```python
from build123d import *

# Parameters (mm, degrees)
BOSS_EXTRUDE1_DEPTH = 12.7
BOSS_EXTRUDE2_DEPTH = 127
BOSS_EXTRUDE3_START = -12.7
SKETCH2_R           = 38.1
SKETCH2_R_2         = 31.75
BOSS_EXTRUDE3_DEPTH = 12.7
BOSS_EXTRUDE4_START = 76.2
BOSS_EXTRUDE4_DEPTH = 76.2


with BuildPart() as part:
    # Sketch1 → Boss-Extrude1 (new body)
    with BuildSketch(Plane(origin=(0, 0, 0), x_dir=(1, 0, 0), z_dir=(0, 1, 0))):
        with BuildLine():
            ThreePointArc((-38.1, 0), (-32.995567884, -19.05), (-19.05, -32.995567884))
            Line((-19.05, -32.995567884), (-15.875, -27.49630657))
            ThreePointArc((-15.875, -27.49630657), (-27.49630657, -15.875), (-31.75, 0))
            Line((-31.75, 0), (-38.1, 0))
        make_face()
        with BuildLine():
            ThreePointArc((-32.995567884, 19.05), (-36.801773982, 9.861005618), (-38.1, 0))
            Line((-38.1, 0), (-31.75, 0))
            ThreePointArc((-31.75, 0), (-30.668144985, 8.217504682), (-27.49630657, 15.875))
            Line((-27.49630657, 15.875), (-32.995567884, 19.05))
        make_face()
        with BuildLine():
            ThreePointArc((0, 38.1), (-19.05, 32.995567884), (-32.995567884, 19.05))
            Line((-32.995567884, 19.05), (-27.49630657, 15.875))
            ThreePointArc((-27.49630657, 15.875), (-15.875, 27.49630657), (0, 31.75))
            Line((0, 31.75), (0, 38.1))
        make_face()
        with BuildLine():
            ThreePointArc((-19.05, -32.995567884), (-9.861005618, -36.801773982), (0, -38.1))
            Line((0, -38.1), (0, -31.75))
            ThreePointArc((0, -31.75), (-8.217504682, -30.668144985), (-15.875, -27.49630657))
            Line((-15.875, -27.49630657), (-19.05, -32.995567884))
        make_face()
        with BuildLine():
            Line((0, -31.75), (0, -38.1))
            ThreePointArc((0, -38.1), (19.05, -32.995567884), (32.995567884, -19.05))
            Line((32.995567884, -19.05), (27.49630657, -15.875))
            ThreePointArc((27.49630657, -15.875), (15.875, -27.49630657), (0, -31.75))
        make_face()
        with BuildLine():
            Line((27.49630657, -15.875), (32.995567884, -19.05))
            ThreePointArc((32.995567884, -19.05), (36.801773982, -9.861005618), (38.1, 0))
            Line((38.1, 0), (31.75, 0))
            ThreePointArc((31.75, 0), (30.668144985, -8.217504682), (27.49630657, -15.875))
        make_face()
        with BuildLine():
            Line((31.75, 0), (38.1, 0))
            ThreePointArc((38.1, 0), (32.995567884, 19.05), (19.05, 32.995567884))
            Line((19.05, 32.995567884), (15.875, 27.49630657))
            ThreePointArc((15.875, 27.49630657), (27.49630657, 15.875), (31.75, 0))
        make_face()
        with BuildLine():
            Line((15.875, 27.49630657), (19.05, 32.995567884))
            ThreePointArc((19.05, 32.995567884), (9.861005618, 36.801773982), (0, 38.1))
            Line((0, 38.1), (0, 31.75))
            ThreePointArc((0, 31.75), (8.217504682, 30.668144985), (15.875, 27.49630657))
        make_face()
    extrude(amount=BOSS_EXTRUDE1_DEPTH)

    # Sketch1_3 → Boss-Extrude2 (add)
    with BuildSketch(Plane(origin=(0, 0, 0), x_dir=(1, 0, 0), z_dir=(0, 1, 0))):
        with BuildLine():
            ThreePointArc((-19.05, -32.995567884), (-9.861005618, -36.801773982), (0, -38.1))
            Line((0, -38.1), (0, -31.75))
            ThreePointArc((0, -31.75), (-8.217504682, -30.668144985), (-15.875, -27.49630657))
            Line((-15.875, -27.49630657), (-19.05, -32.995567884))
        make_face()
        with BuildLine():
            Line((27.49630657, -15.875), (32.995567884, -19.05))
            ThreePointArc((32.995567884, -19.05), (36.801773982, -9.861005618), (38.1, 0))
            Line((38.1, 0), (31.75, 0))
            ThreePointArc((31.75, 0), (30.668144985, -8.217504682), (27.49630657, -15.875))
        make_face()
        with BuildLine():
            Line((15.875, 27.49630657), (19.05, 32.995567884))
            ThreePointArc((19.05, 32.995567884), (9.861005618, 36.801773982), (0, 38.1))
            Line((0, 38.1), (0, 31.75))
            ThreePointArc((0, 31.75), (8.217504682, 30.668144985), (15.875, 27.49630657))
        make_face()
        with BuildLine():
            ThreePointArc((-32.995567884, 19.05), (-36.801773982, 9.861005618), (-38.1, 0))
            Line((-38.1, 0), (-31.75, 0))
            ThreePointArc((-31.75, 0), (-30.668144985, 8.217504682), (-27.49630657, 15.875))
            Line((-27.49630657, 15.875), (-32.995567884, 19.05))
        make_face()
    extrude(amount=BOSS_EXTRUDE2_DEPTH)

    # Sketch2 → Boss-Extrude3 (add)
    with BuildSketch(Plane(origin=(0, 127, 0), x_dir=(1, 0, 0), z_dir=(0, 1, 0)).offset(BOSS_EXTRUDE3_START)):
        with Locations(Location((0, 0, 0), (0, 0, 270))):
            Circle(SKETCH2_R)
        with Locations(Location((0, 0, 0), (0, 0, 270))):
            Circle(SKETCH2_R_2, mode=Mode.SUBTRACT)
    extrude(amount=BOSS_EXTRUDE3_DEPTH)

    # Sketch3 → Boss-Extrude4 (add)
    with BuildSketch(Plane.XZ.offset(BOSS_EXTRUDE4_START)):
        with BuildLine():
            ThreePointArc((36.049475066, 12.330666952), (25.6, 0), (36.049475066, -12.330666952))
            ThreePointArc((36.049475066, -12.330666953), (38.1, 0), (36.049475066, 12.330666953))
        make_face()
        with BuildLine():
            ThreePointArc((34.369685039, 9.2781868), (35.6, 0), (34.369685039, -9.2781868))
            ThreePointArc((34.369685039, -9.2781868), (28.1, 0), (34.369685039, 9.2781868))
        make_face(mode=Mode.SUBTRACT)
    extrude(amount=-BOSS_EXTRUDE4_DEPTH)


solid = part.part
```
Verification items for the finished model (mm, model axes). A direction names the side the tool comes from. Round coordinates to 2 decimals unless told otherwise and drop trailing zeros. Loops run counter-clockwise (first coordinate to the right, second up) from the corner with the lowest first, then second, coordinate; pieces in that order, holes last. Notation, with made-up numbers: (26, -23) -> (63, -23) arc R10 cw to (63, -13) -> close; hole circle Ø3 at (82.5, 30.5). An arc over 180 degrees is marked (long way). Answer as a JSON object with one key per item and string values.
Q1. Go/stop test with flat-tipped pins: P1, Ø1, axis at x = 15.5, y = 86.5, coming from the -Z side; P2, Ø18, axis at x = 13, z = 22.5, coming from the -Y side; P3, Ø11, axis at x = 27, z = -13, coming from the +Y side; P4, Ø1.9, axis at x = 36, y = 55, coming from the -Z side. Record where each tip stops, or that it passes through.
Data:
{"P1": "stops at z = -35.02", "P2": "stops at y = 0", "P3": "stops at y = 127", "P4": "stops at z = 0"}
Q2. Section check D-D (x = 10). Record the boundary of the cut face in (y, z), then the cut area to 3 significant figures.
Data:
{"outline": "(0, -36.76) -> (127, -36.76) -> (127, -30.13) -> (0, -30.13) -> close; (0, 30.13) -> (12.7, 30.13) -> (12.7, 36.76) -> (0, 36.76) -> close; (114.3, 30.13) -> (127, 30.13) -> (127, 36.76) -> (114.3, 36.76) -> close", "area": "1,010 mm2"}
Q3. Section check B-B (x = -24.5). Record the boundary of the cut face in (y, z), then the cut area to 3 significant figures.
Data:
{"outline": "(0, -29.18) -> (12.7, -29.18) -> (12.7, -20.19) -> (0, -20.19) -> close; (0, 20.19) -> (12.7, 20.19) -> (12.7, 29.18) -> (0, 29.18) -> close; (114.3, -29.18) -> (127, -29.18) -> (127, -20.19) -> (114.3, -20.19) -> close; (114.3, 20.19) -> (127, 20.19) -> (127, 29.18) -> (114.3, 29.18) -> close", "area": "456 mm2"}
Q4. Access from +Z, -Z, +X, -X, +Y, -Y to the whole of each face (thin tool, end or side, straight path). Record for faces 4 (the flat face through (-35, 63, 0)), 5 (the flat face through (-30.21, 62.79, -17.44)), 6 (the flat face through (0, 63, -35)), 7 (the cylindrical face through (25.6, -38.6, 0.2)).
Data:
{"face 4": "+Z, -X", "face 5": "-Z, +X", "face 6": "-Z, -X", "face 7": "-X, -Y"}
Q5. Section check C-C (z = 4). Record the boundary of the cut face in (x, y).
Data:
{"outline": "(-37.89, 0) -> (-31.5, 0) -> (-31.5, 12.7) -> (-37.89, 12.7) -> close; (-37.89, 114.3) -> (-31.5, 114.3) -> (-31.5, 127) -> (-37.89, 127) -> close; (26.26, -76.2) -> (28.93, -76.2) -> (28.93, 0) -> (26.26, 0) -> close; (31.5, 0) -> (35.37, 0) -> (35.37, -76.2) -> (37.89, -76.2) -> (37.89, 127) -> (31.5, 127) -> close"}
Q6. Section check A-A (y = 20). Record the boundary of the cut face in (x, z) (3 decimals).
Data:
{"outline": "(-38.1, 0) arc R38.1 ccw to (-32.996, -19.05) -> (-27.496, -15.875) arc R31.75 cw to (-31.75, 0) -> close; (-19.05, 32.996) -> (-15.875, 27.496) arc R31.75 cw to (0, 31.75) -> (0, 38.1) arc R38.1 ccw to start; (0, -38.1) arc R38.1 ccw to (19.05, -32.996) -> (15.875, -27.496) arc R31.75 cw to (0, -31.75) -> close; (27.496, 15.875) arc R31.75 cw to (31.75, 0) -> (38.1, 0) arc R38.1 ccw to (32.996, 19.05) -> close"}
Q7. Scan lines: line 1 (X direction, y = 10, z = -1); line 2 (Y direction, x = -28, z = -22.5); line 3 (X direction, y = -30.5, z = -7.5). Record each from-to range of solid material in increasing order. Write a range as from..to.
Data:
{"line 1": "x = -38.09..-31.73, 31.73..38.09", "line 2": "y = 0..12.7, 114.3..127", "line 3": "x = 28.1..31.49, 34.8..37.35"}
Q8. Draft check along X on faces 1 (the flat face through (-29, 114.3, 16)), 2 (the flat face through (-17.44, 62.79, 30.21)), 3 (the flat face through (33, 0, 0)). Enter one of: pulls with the +X half, pulls with the -X half, needs draft (parallel to the pull), parting line crosses it, or undercut.
Data:
{"face 1": "needs draft", "face 2": "pulls with the -X half", "face 3": "undercut"}
